from build123d import *

# Parameters (mm, degrees)
CROQUIS1_W              = 434
CROQUIS1_H              = 500
SALIENTE_EXTRUIR1_DEPTH = 2
CROQUIS3_W              = 157
CROQUIS3_H              = 90
CORTAR_EXTRUIR2_DEPTH   = 2
REDONDEO1_R             = 5
CORTAR_EXTRUIR3_DEPTH   = 2
REDONDEO2_R             = 20
CROQUIS6_R              = 1.55
CORTAR_EXTRUIR5_DEPTH   = 2
CROQUIS7_R              = 1.55
CORTAR_EXTRUIR6_DEPTH   = 2
CROQUIS8_W              = 20
CROQUIS8_H              = 100
SALIENTE_EXTRUIR2_DEPTH = 2
REDONDEO3_R             = 10
CROQUIS9_R              = 1.55
CORTAR_EXTRUIR7_DEPTH   = 2
CROQUIS10_OUTSIDE_W     = 568.418
CROQUIS10_OUTSIDE_H     = 634.418
CORTAR_EXTRUIR8_DEPTH   = 10
CROQUIS11_W             = 275
CROQUIS11_H             = 1.25
CORTAR_EXTRUIR9_DEPTH   = 2
CROQUIS12_W             = 1
CROQUIS12_H             = 408
SALIENTE_EXTRUIR3_DEPTH = 2


with BuildPart() as part:
    # Croquis1 → Saliente-Extruir1 (new body)
    with BuildSketch(Plane(origin=(0, 0, 0), x_dir=(1, 0, 0), z_dir=(0, 1, 0))):
        with Locations((217, 250)):
            Rectangle(CROQUIS1_W, CROQUIS1_H)
    extrude(amount=SALIENTE_EXTRUIR1_DEPTH)

    # Croquis3 → Cortar-Extruir2 (cut)
    with BuildSketch(Plane.XZ):
        with Locations((78.5, -455)):
            Rectangle(CROQUIS3_W, CROQUIS3_H)
    extrude(amount=-CORTAR_EXTRUIR2_DEPTH, mode=Mode.SUBTRACT)

    # Redondeo1
    redondeo1_edges = [part.edges().sort_by_distance(p)[0] for p in [
        (157, 1, -410),
    ]]
    fillet(redondeo1_edges, radius=REDONDEO1_R)

    # Croquis4 → Cortar-Extruir3 (cut)
    with BuildSketch(Plane.XZ):
        Polygon((30, -20), (394, -20), (394, -233.661541009), (394, -470), (182, -470), (182, -385), (30, -385), align=None)
    extrude(amount=-CORTAR_EXTRUIR3_DEPTH, mode=Mode.SUBTRACT)

    # Redondeo2
    redondeo2_edges = [part.edges().sort_by_distance(p)[0] for p in [
        (30, 1, -385),
        (30, 1, -20),
        (394, 1, -20),
        (394, 1, -470),
        (182, 1, -470),
        (182, 1, -385),
    ]]
    fillet(redondeo2_edges, radius=REDONDEO2_R)

    # Croquis6 → Cortar-Extruir5 (cut)
    with BuildSketch(Plane.XZ):
        with Locations(Location((75, -14, 0), (0, 0, 270))):
            Circle(CROQUIS6_R)
        with Locations(Location((365, -14, 0), (0, 0, 270))):
            Circle(CROQUIS6_R)
        with Locations(Location((288, -476, 0), (0, 0, 270))):
            Circle(CROQUIS6_R)
        with Locations(Location((106, -391, 0), (0, 0, 270))):
            Circle(CROQUIS6_R)
        with Locations(Location((24, -202.5, 0), (0, 0, 270))):
            Circle(CROQUIS6_R)
        with Locations(Location((400, -202.5, 0), (0, 0, 270))):
            Circle(CROQUIS6_R)
    extrude(amount=-CORTAR_EXTRUIR5_DEPTH, mode=Mode.SUBTRACT)

    # Croquis7 → Cortar-Extruir6 (cut)
    with BuildSketch(Plane.XZ):
        with Locations(Location((424.25, -25, 0), (0, 0, 270))):
            Circle(CROQUIS7_R)
        with Locations(Location((424.25, -39, 0), (0, 0, 270))):
            Circle(CROQUIS7_R)
        with Locations(Location((424.25, -475, 0), (0, 0, 270))):
            Circle(CROQUIS7_R)
        with Locations(Location((424.25, -461, 0), (0, 0, 270))):
            Circle(CROQUIS7_R)
        with Locations(Location((424.25, -243, 0), (0, 0, 270))):
            Circle(CROQUIS7_R)
        with Locations(Location((424.25, -257, 0), (0, 0, 270))):
            Circle(CROQUIS7_R)
    extrude(amount=-CORTAR_EXTRUIR6_DEPTH, mode=Mode.SUBTRACT)

    # Croquis8 → Saliente-Extruir2 (add)
    with BuildSketch(Plane.XZ):
        with Locations((40, -205)):
            Rectangle(CROQUIS8_W, CROQUIS8_H)
    extrude(amount=-SALIENTE_EXTRUIR2_DEPTH)

    # Redondeo3
    redondeo3_edges = [part.edges().sort_by_distance(p)[0] for p in [
        (30, 1, -255),
        (30, 1, -155),
    ]]
    fillet(redondeo3_edges, radius=REDONDEO3_R)
    redondeo3_2_edges = [part.edges().sort_by_distance(p)[0] for p in [
        (50, 1, -255),
        (50, 1, -155),
    ]]
    fillet(redondeo3_2_edges, radius=REDONDEO3_R - 0.0001)  # a hair under: the kernel refuses the full size

    # Croquis9 → Cortar-Extruir7 (cut)
    with BuildSketch(Plane.XZ):
        with Locations(Location((42, -165, 0), (0, 0, 270))):
            Circle(CROQUIS9_R)
        with Locations(Location((42, -245, 0), (0, 0, 270))):
            Circle(CROQUIS9_R)
    extrude(amount=-CORTAR_EXTRUIR7_DEPTH, mode=Mode.SUBTRACT)

    # Croquis10 outside → Cortar-Extruir8 (cut)
    with BuildSketch(Plane.XZ):
        with Locations((217, -250)):
            Rectangle(CROQUIS10_OUTSIDE_W, CROQUIS10_OUTSIDE_H)
        with BuildLine():
            Line((1, -409), (152, -409))
            ThreePointArc((152, -409), (156.242640687, -410.757359313), (158, -415))
            Line((158, -415), (158, -499))
            Line((158, -499), (433, -499))
            Line((433, -499), (433, -1))
            Line((433, -1), (1, -1))
            Line((1, -1), (1, -409))
        make_face(mode=Mode.SUBTRACT)
    extrude(amount=-CORTAR_EXTRUIR8_DEPTH, mode=Mode.SUBTRACT)

    # Croquis11 → Cortar-Extruir9 (cut)
    with BuildSketch(Plane.XZ):
        with Locations((295.5, -498.375)):
            Rectangle(CROQUIS11_W, CROQUIS11_H)
    extrude(amount=-CORTAR_EXTRUIR9_DEPTH, mode=Mode.SUBTRACT)

    # Croquis12 → Saliente-Extruir3 (add)
    with BuildSketch(Plane.XZ):
        with Locations((0.5, -205)):
            Rectangle(CROQUIS12_W, CROQUIS12_H)
    extrude(amount=-SALIENTE_EXTRUIR3_DEPTH)


solid = part.part
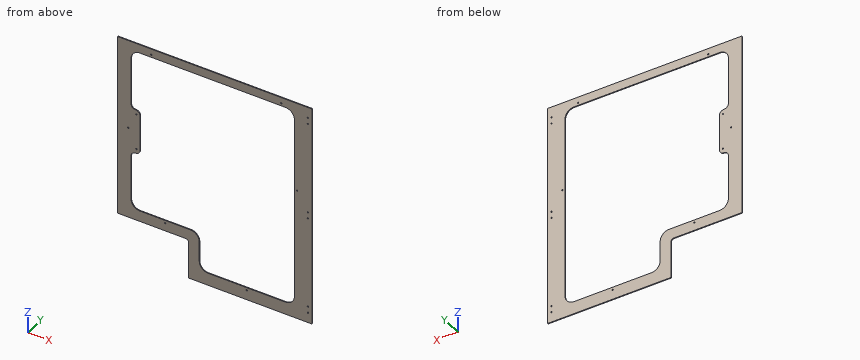
Here's how the part is built. I have some questions about the finished solid (model axes, mm). Round coordinates to 2 decimals unless told otherwise and drop trailing zeros. Write each loop counter-clockwise with the first axis right and the second up, starting at its lowest first coordinate (ties: lowest second). Pieces come first, ordered by that corner, then holes.
1. Suppose I cut it at B-B (y = 1.7). State how many separate pieces and enclosed holes the cut face has, and give its area (3 significant figures).
2. I need wall thicknesses on L1, parallel to Z at x = 75, y = 1.25; L2, parallel to X at y = 1.65, z = -245; L3, parallel to Z at x = 288, y = 1.05. Which ranges of each line are inside material? Lowest first, please.
3. Will these pins go through, and if not, where does the flat tip stop? pin 1 Ø3.5 at (x, z) = (75, -14) entering from +Y; pin 2 Ø1.9 at (x, z) = (424.25, -257) entering from -Y.
4. Suppose I cut it at A-A (z = -184.5). List the corners of the cut face in (x, y) for me, and give its area (3 significant figures).
Answer sheet:
1. separate pieces: 1
1. enclosed holes: 15
1. area: 52,400 mm2
2. L1: z = -409 to -385, -20 to -15.55, -12.45 to -1
2. L2: x = 0 to 40.45, 43.55 to 50, 394 to 433
2. L3: z = -497.75 to -477.55, -474.45 to -470, -20 to -1
3. pin 1: stops at y = 2
3. pin 2: passes through
4. outline: (0, 0) - (50, 0) - (50, 2) - (0, 2) - close; (394, 0) - (433, 0) - (433, 2) - (394, 2) - close
4. area: 178 mm2
